Source: CAD feature listing. Evaluate the final solid. Frame: model axes, mm. Round coordinates to 2 decimals unless told otherwise and drop trailing zeros. Order: outer loops, then holes, each group sorted by start corner. A loop starts at its lowest first (then second) coordinate and runs counter-clockwise, first axis right, second up. Notation, with made-up numbers: (-4.75, 62) -> (50.25, 62) arc R17 ccw to (50.25, 71) -> close; hole circle Ø5 at (67, 74.25). An arc over 180 degrees is marked (long way). Answer as CSV lines item,"result".
from build123d import *

# Parameters (mm, degrees)
SKETCH1_W                   = 70
SKETCH1_H                   = 125
BOSS_EXTRUDE1_DEPTH         = 2
LO_XUYEN_M3_D3_4_DEPTH      = 72.660658663
LO_XUYEN_M3_D3_4_DEPTH_BACK = 72.660658663
SKETCH2_R                   = 1.7
THAN_RANH_DEPTH             = 72.660658663
THAN_RANH_DEPTH_BACK        = 72.660658663
SKETCH3_W                   = 5
SKETCH3_H                   = 15
DAU_RANH_R2_5_DEPTH         = 72.660658663
DAU_RANH_R2_5_DEPTH_BACK    = 72.660658663
SKETCH4_R                   = 2.5


with BuildPart() as part:
    # Sketch1 → Boss-Extrude1 (new body)
    with BuildSketch(Plane.XY):
        Rectangle(SKETCH1_W, SKETCH1_H)
    extrude(amount=-BOSS_EXTRUDE1_DEPTH)

    # Sketch2 → Lo_xuyen_M3_D3_4 (cut, two sides: drawn at the far end of the back side and taken through both)
    with BuildSketch(Plane.XY.offset(-LO_XUYEN_M3_D3_4_DEPTH_BACK)):
        with Locations((-30, -55)):
            Circle(SKETCH2_R)
        with Locations((-30, -37.5)):
            Circle(SKETCH2_R)
        with Locations((-30, 37.5)):
            Circle(SKETCH2_R)
        with Locations((-30, 55)):
            Circle(SKETCH2_R)
        with Locations((30, -55)):
            Circle(SKETCH2_R)
        with Locations((30, -37.5)):
            Circle(SKETCH2_R)
        with Locations((30, 37.5)):
            Circle(SKETCH2_R)
        with Locations((30, 55)):
            Circle(SKETCH2_R)
        with Locations((-12.5, -42.5)):
            Circle(SKETCH2_R)
        with Locations((-12.5, 42.5)):
            Circle(SKETCH2_R)
        with Locations((12.5, -42.5)):
            Circle(SKETCH2_R)
        with Locations((12.5, 42.5)):
            Circle(SKETCH2_R)
    extrude(amount=LO_XUYEN_M3_D3_4_DEPTH + LO_XUYEN_M3_D3_4_DEPTH_BACK, mode=Mode.SUBTRACT)

    # Sketch3 → Than_ranh (cut, two sides: drawn at the far end of the back side and taken through both)
    with BuildSketch(Plane.XY.offset(-THAN_RANH_DEPTH_BACK)):
        with Locations((-25, -17.5)):
            Rectangle(SKETCH3_W, SKETCH3_H)
        with Locations((-25, 17.5)):
            Rectangle(SKETCH3_W, SKETCH3_H)
        with Locations((25, -17.5)):
            Rectangle(SKETCH3_W, SKETCH3_H)
        with Locations((25, 17.5)):
            Rectangle(SKETCH3_W, SKETCH3_H)
    extrude(amount=THAN_RANH_DEPTH + THAN_RANH_DEPTH_BACK, mode=Mode.SUBTRACT)

    # Sketch4 → Dau_ranh_R2_5 (cut, two sides: drawn at the far end of the back side and taken through both)
    with BuildSketch(Plane.XY.offset(-DAU_RANH_R2_5_DEPTH_BACK)):
        with Locations((-25, -25)):
            Circle(SKETCH4_R)
        with Locations((-25, -10)):
            Circle(SKETCH4_R)
        with Locations((-25, 10)):
            Circle(SKETCH4_R)
        with Locations((-25, 25)):
            Circle(SKETCH4_R)
        with Locations((25, -25)):
            Circle(SKETCH4_R)
        with Locations((25, -10)):
            Circle(SKETCH4_R)
        with Locations((25, 10)):
            Circle(SKETCH4_R)
        with Locations((25, 25)):
            Circle(SKETCH4_R)
    extrude(amount=DAU_RANH_R2_5_DEPTH + DAU_RANH_R2_5_DEPTH_BACK, mode=Mode.SUBTRACT)


solid = part.part
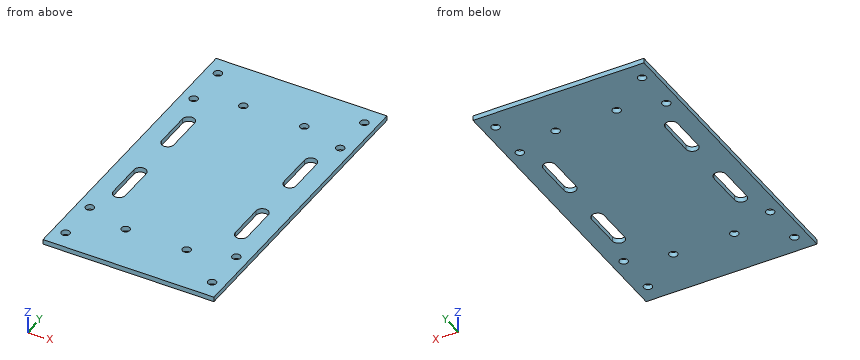
1. Section query D-D on y = 55. Return loops of the section in (x, z).
Results below:
outline,"(-35, -2) -> (-31.7, -2) -> (-31.7, 0) -> (-35, 0) -> close; (-28.3, -2) -> (28.3, -2) -> (28.3, 0) -> (-28.3, 0) -> close; (31.7, -2) -> (35, -2) -> (35, 0) -> (31.7, 0) -> close"
2. Section query B-B on x = -30. Return loops of the section in (y, z).
Results below:
outline,"(-62.5, -2) -> (-56.7, -2) -> (-56.7, 0) -> (-62.5, 0) -> close; (-53.3, -2) -> (-39.2, -2) -> (-39.2, 0) -> (-53.3, 0) -> close; (-35.8, -2) -> (35.8, -2) -> (35.8, 0) -> (-35.8, 0) -> close; (39.2, -2) -> (53.3, -2) -> (53.3, 0) -> (39.2, 0) -> close; (56.7, -2) -> (62.5, -2) -> (62.5, 0) -> (56.7, 0) -> close"
3. Pin query (flat end, axial travel): pin 1 (2 mm diameter, centred on x = 30, y = 37.5, fed in from -Z). Return the tip coordinate at first contact, or that it passes through.
Results below:
pin 1,"through"
4. Section query C-C on z = -1.05. Give the number of separate pieces and of enclosed holes in the cut face, and give its area (3 significant figures).
Results below:
separate pieces,"1"
enclosed holes,"16"
area,"8,260 mm2"
5. Section query A-A on y = 20.5. Return loops of the section in (x, z), and give its area (3 significant figures).
Results below:
outline,"(-35, -2) -> (-27.5, -2) -> (-27.5, 0) -> (-35, 0) -> close; (-22.5, -2) -> (22.5, -2) -> (22.5, 0) -> (-22.5, 0) -> close; (27.5, -2) -> (35, -2) -> (35, 0) -> (27.5, 0) -> close"
area,"120 mm2"
6. Line query: L1, parallel to Y at x = -30, z = -0.85; L2, parallel to X at y = -55, z = -0.4; L3, parallel to Y at x = 12.5, z = -0.6. Output: solid intervals per line, ascending. Write a range as [from, to].
Results below:
L1,"[-62.5, -56.7], [-53.3, -39.2], [-35.8, 35.8], [39.2, 53.3], [56.7, 62.5]"
L2,"[-35, -31.7], [-28.3, 28.3], [31.7, 35]"
L3,"[-62.5, -44.2], [-40.8, 40.8], [44.2, 62.5]"
